Can you work these out from the model? Positions are in its coordinate system, mm. A direction names the side the tool comes from. Coordinates: 2 decimals unless noted, no trailing zeros. Write each loop counter-clockwise with the first axis right and the second up, starting at its lowest first coordinate (ties: lowest second). Pieces come first, ordered by that corner, then holes. Notation, with made-up numbers: (-38.75, -18) -> (8.25, -18) arc R17 ccw to (8.25, 13) -> close; hole circle Ø11 at (68, -34.75). An arc over 180 degrees is marked (long way). Use one line per item in the form item = value.
```python
from build123d import *

# Parameters (mm, degrees)
EXTRUDE020_DEPTH  = 10
CYLINDER133_R     = 2.8
CYLINDER133_DEPTH = 300
CYLINDER134_R     = 2.8
CYLINDER134_DEPTH = 300
EXTRUDE023_DEPTH  = 30
SKETCH037_R       = 93
SKETCH037_R_2     = 11
SKETCH037_R_3     = 15.1
SKETCH037_R_4     = 6.4
EXTRUDE019_DEPTH  = 8
EXTRUDE036_DEPTH  = 100
FILLET008_R       = 5
FILLET009_R       = 2
FILLET010_R       = 5


with BuildPart() as obj1:
    # Sketch038 → Extrude020 (new body)
    with BuildSketch(Plane.XY):
        with BuildLine():
            ThreePointArc((-5, -220), (0, -225), (5, -220))
            Line((5, -220), (5, -212.5))
            ThreePointArc((5, -212.5), (0, -207.5), (-5, -212.5))
            Line((-5, -212.5), (-5, -220))
        make_face()
    extrude(amount=EXTRUDE020_DEPTH)


with BuildPart() as obj1_1:
    # Extrude020 placement: moved
    add(obj1.part.moved(Location((0, 0, -246.5))))


with BuildPart() as cylinder133:
    # Cylinder133 → Cylinder133 (new body)
    with BuildSketch(Plane(origin=(0, 0, 90), x_dir=(1, 0, 0), z_dir=(0, -1, 0))):
        Circle(CYLINDER133_R)
    extrude(amount=CYLINDER133_DEPTH)


with BuildPart() as m4heatsetcuts001:
    # Cylinder134 → Cylinder134 (new body)
    with BuildSketch(Plane(origin=(-150, -150, 90), x_dir=(0, 1, 0), z_dir=(1, 0, 0))):
        Circle(CYLINDER134_R)
    extrude(amount=CYLINDER134_DEPTH)

    # Fusion085: union Cylinder133
    add(cylinder133.part)


with BuildPart() as m4heatsetcuts001_1:
    # Fusion085 placement: moved
    add(m4heatsetcuts001.part.moved(Location((0, 0, -321))))


with BuildPart() as obj2:
    # Sketch041 → Extrude023 (new body)
    with BuildSketch(Plane.XY):
        with BuildLine():
            ThreePointArc((-89.576783, -125), (-93, -150), (-89.576783, -175))
            Line((-89.576783, -175), (-82.286086, -175))
            ThreePointArc((-82.286086, -125), (-86, -150), (-82.286086, -175))
            Line((-89.576783, -125), (-82.286086, -125))
        make_face()
        with BuildLine():
            ThreePointArc((25, -60.423217), (0, -57), (-25, -60.423217))
            Line((-25, -60.423217), (-25, -67.713914))
            ThreePointArc((25, -67.713914), (0, -64), (-25, -67.713914))
            Line((25, -60.423217), (25, -67.713914))
        make_face()
        with BuildLine():
            ThreePointArc((89.576783, -175), (93, -150), (89.576783, -125))
            Line((89.576783, -125), (82.286086, -125))
            ThreePointArc((82.286086, -175), (86, -150), (82.286086, -125))
            Line((89.576783, -175), (82.286086, -175))
        make_face()
        with BuildLine():
            ThreePointArc((-25, -239.576783), (0, -243), (25, -239.576783))
            Line((25, -239.576783), (25, -232.286086))
            ThreePointArc((-25, -232.286086), (0, -236), (25, -232.286086))
            Line((-25, -239.576783), (-25, -232.286086))
        make_face()
    extrude(amount=EXTRUDE023_DEPTH)


with BuildPart() as obj2_1:
    # Extrude023 placement: moved
    add(obj2.part.moved(Location((0, 0, -250))))


with BuildPart() as level5s:
    # Sketch037 → Extrude019 (new body)
    with BuildSketch(Plane.XY):
        with Locations((0, -150)):
            Circle(SKETCH037_R)
        with Locations((-57, -150)):
            Circle(SKETCH037_R_2, mode=Mode.SUBTRACT)
        with Locations((57, -150)):
            Circle(SKETCH037_R_3, mode=Mode.SUBTRACT)
        with Locations((35, -200)):
            Circle(SKETCH037_R_3, mode=Mode.SUBTRACT)
        with Locations((-35, -200)):
            Circle(SKETCH037_R_4, mode=Mode.SUBTRACT)
        with BuildLine():
            ThreePointArc((-3.2, -216.158125), (0, -225), (3.2, -216.158125))
            Line((3.2, -216.158125), (3.2, -212.5))
            ThreePointArc((3.2, -212.5), (0, -209.3), (-3.2, -212.5))
            Line((-3.2, -212.5), (-3.2, -216.158125))
        make_face(mode=Mode.SUBTRACT)
    extrude(amount=EXTRUDE019_DEPTH)


with BuildPart() as level5s_1:
    # Extrude019 placement: moved
    add(level5s.part.moved(Location((0, 0, -250))))

    # Fusion083: union obj2
    add(obj2_1.part)

    # Cut035: cut m4HeatSetCuts001
    add(m4heatsetcuts001_1.part, mode=Mode.SUBTRACT)

    # Cut041: cut obj1
    add(obj1_1.part, mode=Mode.SUBTRACT)


with BuildPart() as fillet010:
    # Sketch054 → Extrude036 (new body)
    with BuildSketch(Plane.XZ):
        Polygon((-20.75, -250), (-12.75, -250), (-12.75, -275.75), (12.75, -275.75), (12.75, -250), (20.75, -250), (20.75, -283.75), (-20.75, -283.75), align=None)
    extrude(amount=EXTRUDE036_DEPTH)


with BuildPart() as fillet010_1:
    # Extrude036 placement: moved
    add(fillet010.part.moved(Location((0, -70, 0))))

    # Fillet008
    fillet008_edges = [fillet010_1.edges().sort_by_distance(p)[0] for p in [
        (20.75, -120, -283.75),
        (-20.75, -120, -283.75),
    ]]
    fillet(fillet008_edges, radius=FILLET008_R)

    # Fillet009
    fillet009_edges = [fillet010_1.edges().sort_by_distance(p)[0] for p in [
        (12.75, -120, -275.75),
        (-12.75, -120, -275.75),
    ]]
    fillet(fillet009_edges, radius=FILLET009_R)

    # Fusion104: union level5s
    add(level5s_1.part)

    # Fillet010
    fillet010_edges = [fillet010_1.edges().sort_by_distance(p)[0] for p in [
        (-20.75, -120, -250),
        (20.75, -120, -250),
    ]]
    fillet(fillet010_edges, radius=FILLET010_R)


solid = fillet010_1.part
```
Q1. Suppose I cut it at B-B (x = 35). Write out the boundary of the cut face in (y, z).
Return value:
outline = (-236.16, -250) -> (-215.1, -250) -> (-215.1, -242) -> (-236.16, -242) -> close; (-184.9, -250) -> (-63.84, -250) -> (-63.84, -242) -> (-184.9, -242) -> close
Q2. Thinking about a two-plate mould opening in X: for faces 1 (the cylindrical face through (65.12, -137.27, -246.06)), 2 (the flat face through (-25, -236, -231)), 3 (the cylindrical face through (-86, -150, -236)), 4 (the flat face through (89, -150, -220)), which applies, released by +X, released by -X, zero draft, split by the parting line, or undercut?
Return value:
face_1 = undercut
face_2 = released by -X
face_3 = undercut
face_4 = zero draft
Q3. Will these pins go through, and if not, where does the flat tip stop? pin 1 (18 mm diameter, centred on x = 35, y = -200, fed in from -Z); pin 2 (3.5 mm diameter, centred on y = -235, z = -226.5, fed in from +X); pin 3 (5 mm diameter, centred on x = 1.5, y = -216, fed in from +Z); pin 4 (11.5 mm diameter, centred on x = 0, y = -220, fed in from +Z).
Return value:
pin_1 = through
pin_2 = 25
pin_3 = -246.5
pin_4 = -242
Q4. For faces 5 (the flat face through (-5, -216, -244)), 6 (the flat face through (0, -119, -275.75)), 7 (the flat face through (-25, -64, -231)), which set-ups out of +Z, -Z, +X, -X, +Y, -Y let a thin tool reach every point of the face, with its end or its side?
Return value:
face_5 = +Z
face_6 = +Y, -Y
face_7 = +Z, -X, +Y, -Y
Q5. Suppose I cut it at C-C (y = -150). Give the number of separate pieces and of enclosed holes in the cut face, then the cut area to 3 significant figures.
Return value:
separate_pieces = 5
enclosed_holes = 1
area = 2,050 mm2
Q6. If I drill on line 1 (Z direction, x = 8, y = -111.5); line 2 (X direction, y = -113, z = -268); line 3 (Y direction, x = 88.5, z = -231), over which ranges is the centre line in solid material (lowest first)? Write a range as from..to.
Return value:
line_1 = -283.75..-275.75, -250..-242
line_2 = -20.75..-12.75, 12.75..20.75
line_3 = -175..-152.8, -147.2..-125
Q7. Suppose I cut it at A-A (z = -268.5). Write out the boundary of the cut face in (x, y).
Return value:
outline = (-20.75, -170) -> (-12.75, -170) -> (-12.75, -70) -> (-20.75, -70) -> close; (12.75, -170) -> (20.75, -170) -> (20.75, -70) -> (12.75, -70) -> close
Q8. Suppose I cut it at D-D (y = -129). Write out the boundary of the cut face in (x, z).
Return value:
outline = (-90.6, -250) -> (-25.75, -250) arc R5 cw to (-20.75, -255) -> (-20.75, -278.75) arc R5 ccw to (-15.75, -283.75) -> (15.75, -283.75) arc R5 ccw to (20.75, -278.75) -> (20.75, -255) arc R5 cw to (25.75, -250) -> (90.6, -250) -> (90.6, -220) -> (83.4, -220) -> (83.4, -242) -> (-83.4, -242) -> (-83.4, -220) -> (-90.6, -220) -> close; hole (-12.75, -273.75) arc R2 ccw to (-10.75, -275.75) -> (10.75, -275.75) arc R2 ccw to (12.75, -273.75) -> (12.75, -250) -> (-12.75, -250) -> close
